from build123d import *

# Parameters (mm, degrees)
ESQUISSE1_R              = 65
BOSS_EXTRU_1_DEPTH       = 2
ESQUISSE2_R              = 1
ENL_V_MAT_EXTRU_1_DEPTH  = 3
ESQUISSE3_R              = 7.5
ENL_V_MAT_EXTRU_2_DEPTH  = 3
ESQUISSE4_R              = 2
ENL_V_MAT_EXTRU_4_DEPTH  = 4
ESQUISSE5_R              = 7.5
BOSS_EXTRU_3_DEPTH       = 4
ESQUISSE6_R              = 2
BOSS_EXTRU_5_DEPTH       = 2
ENL_V_START              = -2
ESQUISSE11_R             = 7.5
ENL_V_MAT_EXTRU_7_DEPTH  = 2
ENL_V_MAT_EXTRU_10_DEPTH = 92.945636112
ENL_V_MAT_EXTRU_11_DEPTH = 10


with BuildPart() as part:
    # Esquisse1 → Boss.-Extru.1 (new body)
    with BuildSketch(Plane(origin=(0, 0, 0), x_dir=(1, 0, 0), z_dir=(0, 1, 0))):
        with Locations(Location((0, 0, 0), (0, 0, 270))):
            Circle(ESQUISSE1_R)
    extrude(amount=BOSS_EXTRU_1_DEPTH)

    # Esquisse2 → Enlèv. mat.-Extru.1 (cut)
    with BuildSketch(Plane(origin=(0, 2, 0), x_dir=(1, 0, 0), z_dir=(0, 1, 0))):
        with Locations(Location((-53.47585562, 32.350932996, 0), (0, 0, 270))):
            Circle(ESQUISSE2_R)
        with Locations(Location((-54.754657621, -30.135982958, 0), (0, 0, 270))):
            Circle(ESQUISSE2_R)
        with Locations(Location((-1.278802001, -62.486915954, 0), (0, 0, 270))):
            Circle(ESQUISSE2_R)
        with Locations(Location((53.47585562, -32.350932996, 0), (0, 0, 270))):
            Circle(ESQUISSE2_R)
        with Locations(Location((54.754657621, 30.135982958, 0), (0, 0, 270))):
            Circle(ESQUISSE2_R)
        with Locations(Location((1.278802001, 62.486915954, 0), (0, 0, 270))):
            Circle(ESQUISSE2_R)
    extrude(amount=-ENL_V_MAT_EXTRU_1_DEPTH, mode=Mode.SUBTRACT)

    # Esquisse3 → Enlèv. mat.-Extru.2 (cut)
    with BuildSketch(Plane(origin=(0, 2, 0), x_dir=(1, 0, 0), z_dir=(0, 1, 0))):
        with Locations(Location((0, 0, 0), (0, 0, 270))):
            Circle(ESQUISSE3_R)
    extrude(amount=-ENL_V_MAT_EXTRU_2_DEPTH, mode=Mode.SUBTRACT)

    # Esquisse4 → Enlèv. mat.-Extru.4 (cut)
    with BuildSketch(Plane(origin=(0, 2, 0), x_dir=(1, 0, 0), z_dir=(0, 1, 0))):
        with Locations(Location((0, 33.5, 0), (0, 0, 270))):
            Circle(ESQUISSE4_R)
        with Locations(Location((29.011851027, 16.75, 0), (0, 0, 270))):
            Circle(ESQUISSE4_R)
        with Locations(Location((29.011851027, -16.75, 0), (0, 0, 270))):
            Circle(ESQUISSE4_R)
        with Locations(Location((0, -33.5, 0), (0, 0, 270))):
            Circle(ESQUISSE4_R)
        with Locations(Location((-29.011851027, -16.75, 0), (0, 0, 270))):
            Circle(ESQUISSE4_R)
        with Locations(Location((-29.011851027, 16.75, 0), (0, 0, 270))):
            Circle(ESQUISSE4_R)
    extrude(amount=-ENL_V_MAT_EXTRU_4_DEPTH, mode=Mode.SUBTRACT)

    # Esquisse5 → Boss.-Extru.3 (add)
    with BuildSketch(Plane(origin=(0, 2, 0), x_dir=(1, 0, 0), z_dir=(0, 1, 0))):
        with Locations(Location((0, 0, 0), (0, 0, 270))):
            Circle(ESQUISSE5_R)
    extrude(amount=-BOSS_EXTRU_3_DEPTH)

    # Esquisse6 → Boss.-Extru.5 (add)
    with BuildSketch(Plane(origin=(0, 2, 0), x_dir=(1, 0, 0), z_dir=(0, 1, 0))):
        with Locations((-29.011851027, 16.75)):
            Circle(ESQUISSE6_R)
        with Locations((29.011851027, 16.75)):
            Circle(ESQUISSE6_R)
        with Locations((29.011851027, -16.75)):
            Circle(ESQUISSE6_R)
        with Locations((0, -33.5)):
            Circle(ESQUISSE6_R)
        with Locations((-29.011851027, -16.75)):
            Circle(ESQUISSE6_R)
        with Locations((0, 33.5)):
            Circle(ESQUISSE6_R)
    extrude(amount=-BOSS_EXTRU_5_DEPTH)

    # Esquisse11 → Enlèv. mat.-Extru.7 (cut)
    with BuildSketch(Plane(origin=(0, -2, 0), x_dir=(-1, 0, 0), z_dir=(0, -1, 0)).offset(ENL_V_START)):
        Circle(ESQUISSE11_R)
    extrude(amount=ENL_V_MAT_EXTRU_7_DEPTH, mode=Mode.SUBTRACT)

    # Esquisse13 → Enlèv. mat.-Extru.10 (cut, through all)
    with BuildSketch(Plane(origin=(0, 0, 0), x_dir=(-1, 0, 0), z_dir=(0, -1, 0))):
        with BuildLine():
            Line((-17.713203436, -3.713203436), (-21.213203436, -3.713203436))
            Line((-21.213203436, -3.713203436), (-21.213203436, -38.713203436))
            Line((-21.213203436, -38.713203436), (-17.713203436, -38.713203436))
            Line((-17.713203436, -38.713203436), (-10.536125184, -38.713203436))
            ThreePointArc((-10.536125184, -38.713203436), (-3.336820913, -31.247392387), (-0.713203436, -21.213203436))
            ThreePointArc((-0.713203436, -21.213203436), (-3.336820913, -11.179014484), (-10.536125184, -3.713203436))
            Line((-10.536125184, -3.713203436), (-17.713203436, -3.713203436))
        make_face()
        with BuildLine():
            Line((-21.213203436, -38.713203436), (-21.213203436, -3.713203436))
            Line((-21.213203436, -3.713203436), (-24.713203436, -3.713203436))
            Line((-24.713203436, -3.713203436), (-31.890281688, -3.713203436))
            ThreePointArc((-31.890281688, -3.713203436), (-41.713203436, -21.213203436), (-31.890281688, -38.713203436))
            Line((-31.890281688, -38.713203436), (-24.713203436, -38.713203436))
            Line((-24.713203436, -38.713203436), (-21.213203436, -38.713203436))
        make_face()
        with BuildLine():
            Line((-21.213203436, -3.713203436), (-21.213203436, -0.713203436))
            ThreePointArc((-21.213203436, -0.713203436), (-22.969662591, -0.788589578), (-24.713203436, -1.014193559))
            Line((-24.713203436, -1.014193559), (-24.713203436, -3.713203436))
            Line((-24.713203436, -3.713203436), (-21.213203436, -3.713203436))
        make_face()
        with BuildLine():
            ThreePointArc((-17.713203436, -1.014193559), (-19.45674428, -0.788589578), (-21.213203436, -0.713203436))
            Line((-21.213203436, -0.713203436), (-21.213203436, -3.713203436))
            Line((-21.213203436, -3.713203436), (-17.713203436, -3.713203436))
            Line((-17.713203436, -3.713203436), (-17.713203436, -1.014193559))
        make_face()
        with BuildLine():
            Line((-17.713203436, -38.713203436), (-21.213203436, -38.713203436))
            Line((-21.213203436, -38.713203436), (-21.213203436, -41.713203436))
            ThreePointArc((-21.213203436, -41.713203436), (-19.45674428, -41.637817293), (-17.713203436, -41.412213312))
            Line((-17.713203436, -41.412213312), (-17.713203436, -38.713203436))
        make_face()
        with BuildLine():
            Line((-21.213203436, -41.713203436), (-21.213203436, -38.713203436))
            Line((-21.213203436, -38.713203436), (-24.713203436, -38.713203436))
            Line((-24.713203436, -38.713203436), (-24.713203436, -41.412213312))
            ThreePointArc((-24.713203436, -41.412213312), (-22.969662591, -41.637817293), (-21.213203436, -41.713203436))
        make_face()
    extrude(amount=-ENL_V_MAT_EXTRU_10_DEPTH, mode=Mode.SUBTRACT)

    # Esquisse14 → Enlèv. mat.-Extru.11 (cut)
    with BuildSketch(Plane(origin=(0, 0, 0), x_dir=(-1, 0, 0), z_dir=(0, -1, 0))):
        with BuildLine():
            Line((24, -32.5), (24, 32.5))
            ThreePointArc((24, 32.5), (25, 33.5), (26, 32.5))
            Line((26, 32.5), (26, -32.5))
            ThreePointArc((26, -32.5), (25, -33.5), (24, -32.5))
        make_face()
        with BuildLine():
            Line((31.003124215, -32.5), (31.003124215, 32.5))
            ThreePointArc((31.003124215, 32.5), (32.003124215, 33.5), (33.003124215, 32.5))
            Line((33.003124215, 32.5), (33.003124215, -32.5))
            ThreePointArc((33.003124215, -32.5), (32.003124215, -33.5), (31.003124215, -32.5))
        make_face()
        with BuildLine():
            Line((16.996875785, -32.5), (16.996875785, 32.5))
            ThreePointArc((16.996875785, 32.5), (17.996875785, 33.5), (18.996875785, 32.5))
            Line((18.996875785, 32.5), (18.996875785, -32.5))
            ThreePointArc((18.996875785, -32.5), (17.996875785, -33.5), (16.996875785, -32.5))
        make_face()
    extrude(amount=-ENL_V_MAT_EXTRU_11_DEPTH, mode=Mode.SUBTRACT)


solid = part.part
The listing builds one solid part. Answer for the finished solid, in the listing's coordinates (mm). Round coordinates to 2 decimals unless told otherwise and drop trailing zeros. Write each loop counter-clockwise with the first axis right and the second up, starting at its lowest first coordinate (ties: lowest second). Pieces come first, ordered by that corner, then holes. Notation, with made-up numbers: M 58,6.25 L 101,6.25 A28 ccw 101,29.25 Z; hole C 4,37 d5. An arc over 180 degrees is marked long. Write each question's results on one line, items separated by ' | '. Start each with the question number.
(1) Find the intervals of material crossed by line 1 (X direction, y = 0.2, z = 0); line 2 (X direction, y = 1.25, z = 9); line 3 (X direction, y = 1.9, z = 10), in increasing order.
(2) The part is cut by section A-A, the plane z = -22. Write down the section's boundary in (x, y), and give its area (3 significant figures).
(3) The part is cut by section B-B, the plane y = 1.25. Give the number of separate pieces and of enclosed holes in the cut face, and give its area (3 significant figures).
(4) The part is cut by section D-D, the plane z = 43.5. Write down the section's boundary in (x, y), and give its area (3 significant figures).
(5) Determine the mould class of faces 1 (the cylindrical face through (19.52, 0.99, 62)), 2 (the cylindrical face through (41.71, 0.99, 20.92)), 3 (the flat face through (1, 0, -1)) for opening direction X: +X half, -X half, draft (parallel to the pull), parting line (faces both ways), or undercut.
(6) The part is cut by section C-C, the plane x = -36.5. Write down the section's boundary in (y, z), and give its area (3 significant figures).
(7) Each of these flat-tipped pins is pushed along its axis until it touches: P1, Ø0.6, axis at y = 1.5, z = -1.5, coming from the +X side; P2, Ø1, axis at x = 13, y = 1.5, coming from the -Z side; P3, Ø1, axis at y = 1, z = 8.5, coming from the -X side; P4, Ø1.6, axis at x = 1.28, z = -62.49, coming from the +Y side (3 decimals). Where does it stop, or does it pass through?
Worked answers:
1) line 1: x = -65 to -33, -31 to -26, -24 to -19, -17 to 65 | line 2: x = -64.37 to -33, -31 to -26, -24 to -19, -17 to 4.75, 37.68 to 64.37 | line 3: x = -64.23 to -33, -31 to -26, -24 to -19, -17 to 4.05, 38.37 to 64.23
2) outline: M -61.16,0 L -33,0 L -33,2 L -61.16,2 Z; M -31,0 L -26,0 L -26,2 L -31,2 Z; M -24,0 L -19,0 L -19,2 L -24,2 Z; M -17,0 L 61.16,0 L 61.16,2 L -17,2 Z | area: 233 mm²
3) separate pieces: 1 | enclosed holes: 10 | area: 11,600 mm²
4) outline: M -48.3,0 L 48.3,0 L 48.3,2 L -48.3,2 Z | area: 193 mm²
5) face 1: parting line | face 2: undercut | face 3: draft
6) outline: M 0,-53.78 L 2,-53.78 L 2,53.78 L 0,53.78 Z | area: 215 mm²
7) P1: stops at x = 64.99 | P2: stops at z = -63.79 | P3: stops at x = -64.51 | P4: passes through
